from build123d import *

# Parameters (mm, degrees)
SKETCH_1_W                = 52
SKETCH_1_H                = 30
EXTRUDE_1_DEPTH           = 22
SKETCH_2_W                = 30
SKETCH_2_H                = 2
CUT_EXTRUDE_1_DEPTH       = 64.937469453
EXTRUDE_2_DEPTH           = 4
SKETCH_4_W                = 5
SKETCH_4_H                = 16
EXTRUDE_3_DEPTH           = 5
HOLE_WIZARD_4_0_4_1_D     = 4
HOLE_WIZARD_4_0_4_1_DEPTH = 6
HOLE_WIZARD_M81_D         = 9.728
HOLE_WIZARD_M81_DEPTH     = 33
HOLE_WIZARD_2_0_2_1_D     = 2
HOLE_WIZARD_2_0_2_1_DEPTH = 2
FILLET_1_R                = 2
CHAMFER_1_SIZE            = 1
CHAMFER_2_SIZE            = 0.5
FILLET_2_R                = 0.5


with BuildPart() as part:
    # Эскиз1 → Бобышка-Вытянуть1 (new body)
    with BuildSketch(Plane(origin=(0, 22, 0), x_dir=(1, 0, 0), z_dir=(0, 1, 0))):
        with Locations((-26, 15)):
            Rectangle(SKETCH_1_W, SKETCH_1_H)
    extrude(amount=-EXTRUDE_1_DEPTH)

    # Эскиз2 → Вырез-Вытянуть1 (cut, through all)
    with BuildSketch(Plane.XZ):
        with Locations((-37, -1)):
            Rectangle(SKETCH_2_W, SKETCH_2_H)
    extrude(amount=-CUT_EXTRUDE_1_DEPTH, mode=Mode.SUBTRACT)

    # Эскиз3 → Бобышка-Вытянуть2 (add)
    with BuildSketch(Plane.ZY.offset(52)):
        Polygon((-14.25, 17.495190528), (-10.5, 11), (-14.25, 4.504809472), (-21.75, 4.504809472), (-25.5, 11), (-21.75, 17.495190528), align=None)
    extrude(amount=EXTRUDE_2_DEPTH)

    # Эскиз4 → Бобышка-Вытянуть3 (add)
    with BuildSketch(Plane.XY.offset(-2)):
        with Locations((-44.5, 11)):
            Rectangle(SKETCH_4_W, SKETCH_4_H)
    extrude(amount=EXTRUDE_3_DEPTH)

    # Диаметр отверстия Ø4.0 (4)1
    with Locations(Plane(origin=(0, 0, 0), x_dir=(0, 0, -1), z_dir=(1, 0, 0))):
        with Locations((4, 3), (4, 19)):
            Hole(HOLE_WIZARD_4_0_4_1_D / 2, depth=HOLE_WIZARD_4_0_4_1_DEPTH)

    # Отверстие с зазором M81
    with Locations(Plane(origin=(0, 0, -30), x_dir=(-1, 0, 0), z_dir=(0, 0, -1))):
        with Locations((8, 11)):
            Hole(HOLE_WIZARD_M81_D / 2, depth=HOLE_WIZARD_M81_DEPTH)

    # Диаметр отверстия Ø2.0 (2)1
    with Locations(Plane.XY.offset(3)):
        with Locations((-44.5, 14), (-44.5, 8)):
            Hole(HOLE_WIZARD_2_0_2_1_D / 2, depth=HOLE_WIZARD_2_0_2_1_DEPTH)

    # Эскиз11 → Диаметр отверстия Ø8.0 (8)1 (revolve, cut)
    with BuildSketch(Plane(origin=(-56, 11, -18), x_dir=(0, 0, 1), z_dir=(0, 1, 0))):
        Polygon((0, 0), (0, 2), (4, 2), (4, 1), (5, 0), align=None)
    revolve(axis=Axis((-62.35, 11, -18), (1, 0, 0)), mode=Mode.SUBTRACT)

    # Скругление1
    fillet_1_edges = [part.edges().sort_by_distance(p)[0] for p in [
        (-52, 0, -16),
        (-26, 0, -30),
        (-52, 11, -30),
        (-26, 22, -30),
        (-52, 22, -16),
        (-11, 22, 0),
        (-11, 0, 0),
        (-54, 17.495190528, -21.75),
        (-54, 11, -25.5),
        (-54, 17.495190528, -14.25),
        (-54, 11, -10.5),
        (-54, 4.504809472, -14.25),
        (-54, 4.504809472, -21.75),
    ]]
    fillet(fillet_1_edges, radius=FILLET_1_R)

    # Фаска1
    chamfer_1_edges = [part.edges().sort_by_distance(p)[0] for p in [
        (-12.864, 11, 0),
        (-12.864, 11, -30),
    ]]
    chamfer(chamfer_1_edges, length=CHAMFER_1_SIZE)

    # Фаска2
    chamfer_2_edges = [part.edges().sort_by_distance(p)[0] for p in [
        (0, 19, -6),
        (0, 3, -6),
    ]]
    chamfer(chamfer_2_edges, length=CHAMFER_2_SIZE)

    # Скругление2
    fillet_2_edges = [part.edges().sort_by_distance(p)[0] for p in [
        (-56, 14.247595264, -23.625),
        (-56, 17.495190528, -18),
        (-56, 7.752404736, -23.625),
        (-56, 4.504809472, -18),
        (-56, 7.752404736, -12.375),
        (-56, 14.247595264, -12.375),
        (-56, 4.772758664, -21.595299462),
        (-56, 4.772758664, -14.404700538),
        (-56, 11, -10.809401077),
        (-56, 17.227241336, -14.404700538),
        (-56, 11, -25.190598923),
        (-56, 17.227241336, -21.595299462),
    ]]
    fillet(fillet_2_edges, radius=FILLET_2_R)


solid = part.part
Model file for the job. Use its own axes, mm. A direction names the side the tool comes from. Coordinates: 2 decimals unless noted, no trailing zeros. Order: outer loops, then holes, each group sorted by start corner. A loop starts at its lowest first (then second) coordinate and runs counter-clockwise, first axis right, second up. Notation, with made-up numbers: M -32,67 L 3,67 A29 cw 3,89 Z; hole C 69.5,11 d10. An arc over 180 degrees is marked long. Return JSON: item names as keys, results as strings.
1. Drill centre lines: probe 1 along Y at (x, z) = (-2.5, -4); probe 2 along Y at (x, z) = (-44.5, 2.1); probe 3 along Y at (x, z) = (-3.7, -4). Where is each one in solid material? Low to high.
Ans:
{"probe 1": "0 to 1, 5 to 17, 21 to 22", "probe 2": "3 to 7, 9 to 13, 15 to 19", "probe 3": "0 to 1, 5 to 8.73, 13.27 to 17, 21 to 22"}
2. Saw through at B-B (x = -8). Give the cut face in (y, z), and give its area (3 significant figures).
Ans:
{"outline": "M 0,-28 A2 ccw 2,-30 L 5.14,-30 L 6.14,-29 L 6.14,-1 L 5.14,0 L 2,0 A2 ccw 0,-2 Z; M 15.86,-29 L 16.86,-30 L 20,-30 A2 ccw 22,-28 L 22,-2 A2 ccw 20,0 L 16.86,0 L 15.86,-1 Z", "area": "363 mm^2"}
3. Flat gauge pins, fed straight in: pin 1 (2.5 mm diameter, centred on y = 11.5, z = -18.5, fed in from -X); pin 2 (10 mm diameter, centred on x = -10.5, y = 6, fed in from +Z); pin 3 (6.5 mm diameter, centred on y = 19, z = -4, fed in from -X); pin 4 (8 mm diameter, centred on x = -8, y = 11, fed in from -Z). Where does each tip first touch, or does it go through?
Ans:
{"pin 1": "x = -54", "pin 2": "z = 0", "pin 3": "x = -52", "pin 4": "through"}
4. Saw through at D-D (x = -23). Give the cut face in (y, z), and give its area (3 significant figures).
Ans:
{"outline": "M 0,-28 A2 ccw 2,-30 L 20,-30 A2 ccw 22,-28 L 22,-2 L 0,-2 Z", "area": "614 mm^2"}
5. Tool access for faces 1 (the face through (-3.3, 1.8, -5.6)), 2 (the face through (-45, 19, 0)), 3 (the face through (-54, 17.495, -18)), 4 (the face through (-42, 11, 0)): list every direction of +Z, -Z, +X, -X, +Y, -Y with a clear straight run to the whole face (end or side of a thin tool).
Ans:
{"face 1": "+X", "face 2": "+Z, -X, +Y", "face 3": "+Z, -Z, -X, +Y", "face 4": "+Z, +Y, -Y"}
6. Saw through at A-A (z = -18). Give the cut face in (x, y).
Ans:
{"outline": "M -56,5 A0.5 ccw -55.5,4.5 L -52,4.5 L -52,2 A2 ccw -50,0 L 0,0 L 0,22 L -50,22 A2 ccw -52,20 L -52,17.5 L -55.5,17.5 A0.5 ccw -56,17 L -56,16 L -55,15 L -54,15 L -54,7 L -55,7 L -56,6 Z; hole C -8,11 d9.73"}
7. Saw through at C-C (z = -4). Give the cut face in (x, y), and give its area (3 significant figures).
Ans:
{"outline": "M -52,2 A2 ccw -50,0 L 0,0 L 0,0.5 L -0.5,1 L -6,1 L -6,5 L -0.5,5 L 0,5.5 L 0,16.5 L -0.5,17 L -6,17 L -6,21 L -0.5,21 L 0,21.5 L 0,22 L -50,22 A2 ccw -52,20 Z; hole C -8,11 d9.73", "area": "1,020 mm^2"}
8. Pull direction X, two halves, no side cores. Call faces 5 (the face through (-53.73, 14.22, -23.64)), 6 (the face through (-56, 15, -14)), 7 (the face through (-44, 14, 1)): +X half, -X half, draft (parallel to the pull), parting line (faces both ways), or undercut.
Ans:
{"face 5": "draft", "face 6": "-X half", "face 7": "undercut"}
